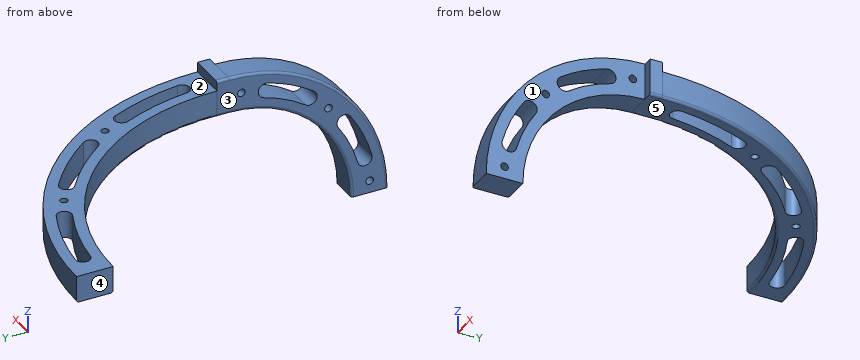
```python
from build123d import *

# Parameters (mm, degrees)
EXTRUDE_1_DEPTH     = 15
SKETCH_2_W          = 15
SKETCH_2_H          = 15
EXTRUDE_2_DEPTH     = 5
EXTRUDE_3_DEPTH     = 15
SKETCH_4_R          = 1.55
CUT_EXTRUDE_1_DEPTH = 163.095650774
SKETCH_5_R          = 1.55
CUT_EXTRUDE_2_DEPTH = 157.68439616
CUT_EXTRUDE_3_DEPTH = 4
CUT_EXTRUDE_START   = -4
CUT_EXTRUDE_4_DEPTH = 4
FILLET_1_R          = 1


with BuildPart() as part:
    # 草图1 → 凸台-拉伸1 (new body)
    with BuildSketch(Plane.XY):
        with BuildLine():
            Line((90, 0), (105, 0))
            ThreePointArc((105, 0), (74.246212025, 74.246212025), (0, 105))
            Line((0, 105), (0, 90))
            ThreePointArc((0, 90), (63.639610307, 63.639610307), (90, 0))
        make_face()
    extrude(amount=EXTRUDE_1_DEPTH)

    # 草图2 → 凸台-拉伸2 (add)
    with BuildSketch(Plane.XZ):
        with Locations((97.5, 7.5)):
            Rectangle(SKETCH_2_W, SKETCH_2_H)
    extrude(amount=EXTRUDE_2_DEPTH)

    # 草图3 → 凸台-拉伸3 (add)
    with BuildSketch(Plane(origin=(105, 0, 0), x_dir=(0, 0, -1), z_dir=(1, 0, 0))):
        with BuildLine():
            Line((50, -55), (50, -70))
            ThreePointArc((50, -70), (4.038059223, -50.961940777), (-15, -5))
            Line((-15, -5), (0, -5))
            ThreePointArc((0, -5), (14.644660941, -40.355339059), (50, -55))
        make_face()
    extrude(amount=-EXTRUDE_3_DEPTH)

    # 草图4 → 切除-拉伸1 (cut, through all)
    with BuildSketch(Plane.XY.offset(15)):
        with Locations((84.437476869, 48.75)):
            Circle(SKETCH_4_R)
        with Locations((48.75, 84.437476869)):
            Circle(SKETCH_4_R)
        with BuildLine():
            ThreePointArc((40.593936087, 91.936838933), (26.011314033, 97.075545542), (10.813039575, 99.916606103))
            ThreePointArc((10.813039575, 99.916606103), (7.507677018, 97.256798147), (10.167484974, 93.951435589))
            ThreePointArc((10.167484974, 93.951435589), (24.458399762, 91.279990584), (38.170417515, 86.448072429))
            ThreePointArc((38.170417515, 86.448072429), (42.126560053, 87.980696395), (40.593936087, 91.936838933))
        make_face()
        with BuildLine():
            ThreePointArc((81.123799357, 59.322670016), (71.064231509, 71.064231509), (59.322670016, 81.123799357))
            ThreePointArc((59.322670016, 81.123799357), (55.130238094, 80.473019377), (55.781018075, 76.280587456))
            ThreePointArc((55.781018075, 76.280587456), (66.821590822, 66.821590822), (76.280587456, 55.781018075))
            ThreePointArc((76.280587456, 55.781018075), (80.473019377, 55.130238094), (81.123799357, 59.322670016))
        make_face()
        with BuildLine():
            ThreePointArc((99.916606103, 10.813039575), (97.075545542, 26.011314033), (91.936838933, 40.593936087))
            ThreePointArc((91.936838933, 40.593936087), (87.980696395, 42.126560053), (86.448072429, 38.170417515))
            ThreePointArc((86.448072429, 38.170417515), (91.279990584, 24.458399762), (93.951435589, 10.167484974))
            ThreePointArc((93.951435589, 10.167484974), (97.256798147, 7.507677018), (99.916606103, 10.813039575))
        make_face()
    extrude(amount=-CUT_EXTRUDE_1_DEPTH, mode=Mode.SUBTRACT)

    # 草图5 → 切除-拉伸2 (cut, through all)
    with BuildSketch(Plane(origin=(105, 0, 0), x_dir=(0, 0, -1), z_dir=(1, 0, 0))):
        with Locations((44.969401847, -62.5)):
            Circle(SKETCH_5_R)
        with Locations((9.341360082, -45.658639918)):
            Circle(SKETCH_5_R)
        with Locations((-7.28119514, -10.011455208)):
            Circle(SKETCH_5_R)
        with BuildLine():
            ThreePointArc((-8.432245014, -20.681924073), (-4.831621116, -30.568404835), (0.427426106, -39.681550102))
            ThreePointArc((0.427426106, -39.681550102), (4.605316552, -40.419947976), (5.343714426, -36.24205753))
            ThreePointArc((5.343714426, -36.24205753), (0.606225607, -28.032695265), (-2.637311624, -19.126691933))
            ThreePointArc((-2.637311624, -19.126691933), (-6.312394389, -17.006841308), (-8.432245014, -20.681924073))
        make_face()
        with BuildLine():
            ThreePointArc((15.318449898, -54.572573894), (24.431595165, -59.831621116), (34.318075927, -63.432245014))
            ThreePointArc((34.318075927, -63.432245014), (37.993158692, -61.312394389), (35.873308067, -57.637311624))
            ThreePointArc((35.873308067, -57.637311624), (26.967304735, -54.393774393), (18.75794247, -49.656285574))
            ThreePointArc((18.75794247, -49.656285574), (14.580052024, -50.394683448), (15.318449898, -54.572573894))
        make_face()
    extrude(amount=-CUT_EXTRUDE_2_DEPTH, mode=Mode.SUBTRACT)

    # 草图6 → 切除-拉伸3 (cut)
    with BuildSketch(Plane(origin=(105, 0, 0), x_dir=(0, 0, -1), z_dir=(1, 0, 0))):
        with BuildLine():
            Line((50, -55), (50, -70))
            ThreePointArc((50, -70), (4.038059223, -50.961940777), (-15, -5))
            Line((-15, -5), (0, -5))
            ThreePointArc((0, -5), (14.644660941, -40.355339059), (50, -55))
        make_face()
    extrude(amount=-CUT_EXTRUDE_3_DEPTH, mode=Mode.SUBTRACT)

    # 草图7 → 切除-拉伸4 (cut)
    with BuildSketch(Plane.XY.offset(15).offset(CUT_EXTRUDE_START)):
        with BuildLine():
            Line((0, 105), (0, 90))
            ThreePointArc((0, 90), (63.639610307, 63.639610307), (90, 0))
            Line((90, 0), (105, 0))
            ThreePointArc((105, 0), (74.246212025, 74.246212025), (0, 105))
        make_face()
    extrude(amount=CUT_EXTRUDE_4_DEPTH, mode=Mode.SUBTRACT)

    # 圆角1
    fillet_1_edges = [part.edges().sort_by_distance(p)[0] for p in [
        (90, -2.5, 15),
        (90, -2.5, 0),
        (105, -2.5, 0),
        (90, -40.355339059, -14.644660941),
        (90, -50.961940777, -4.038059223),
        (63.639610307, 63.639610307, 0),
        (74.246212025, 74.246212025, 0),
    ]]
    fillet(fillet_1_edges, radius=FILLET_1_R)


solid = part.part
```
Can you work these out from the model? Positions are in its coordinate system, mm. Face numbers are marked on the shaded views. A direction names the side the tool comes from. Give positions to 0.01 mm unless a question says otherwise; leave off trailing zeros. Write item = value, one per line. Start each with the question number.
1. On a 3-axis mill with a long thin cutter (end or side, diameter ignored), from which of +Z, -Z, +X, -X, +Y, -Y can I reach the whole of each face in a straight line? I mean the marked faces 1, 2, 3, 4 and 5. Say none if no direction works.
2. For pin 1 (10 mm diameter, centred on x = 84, y = 62, fed in from +Z); pin 2 (12 mm diameter, centred on y = -33.5, z = -0.5, fed in from +X); pin 3 (12 mm diameter, centred on x = 79, z = -13, fed in from -Y); pin 4 (2 mm diameter, centred on x = 99.5, z = 13.5, fed in from +Y), each with a flat end and sliding along its axis, tell me the tip position at first contact or that it passes through.
3. Please list where these lines run through material, in increasing order: line 1 (Y direction, x = 97, z = -5.5); line 2 (Y direction, x = 48, z = 8); line 3 (X direction, y = 79.5, z = 10).
Worked answers:
q1.face_1 = +Z, -Z, +X, -Y
q1.face_2 = +Z, +X, -X, +Y
q1.face_3 = +Z, -Z, -X, -Y
q1.face_4 = +Z, -Z, -X, +Y, -Y
q1.face_5 = -Z, +X, -X, +Y
q2.pin_1 = 11
q2.pin_2 = 101
q2.pin_3 = through
q2.pin_4 = 0
q3.line_1 = -52.38 to -39.43, -36.49 to -27.8
q3.line_2 = 76.13 to 83.08, 85.79 to 93.39
q3.line_3 = 42.19 to 54.66, 61.48 to 68.59
